The figure shows three views and two pictorial views of one solid part (mm, origin at its lowest corner). Answer the questions. A direction names the side the tool comes from. Give positions to 0.01 mm unless a question says otherwise; leave off trailing zeros. Write each loop counter-clockwise with the first axis right and the second up, starting at its lowest first coordinate (ties: lowest second). Pieces come first, ordered by that corner, then holes. Notation, with made-up numbers: M -35.5,-19.5 L -25.5,-19.5 A24 cw -25.5,18.5 Z; hole C 60,41 d1. An arc over 180 degrees is marked long. Answer as CSV lines item,"result". Start each with the question number.
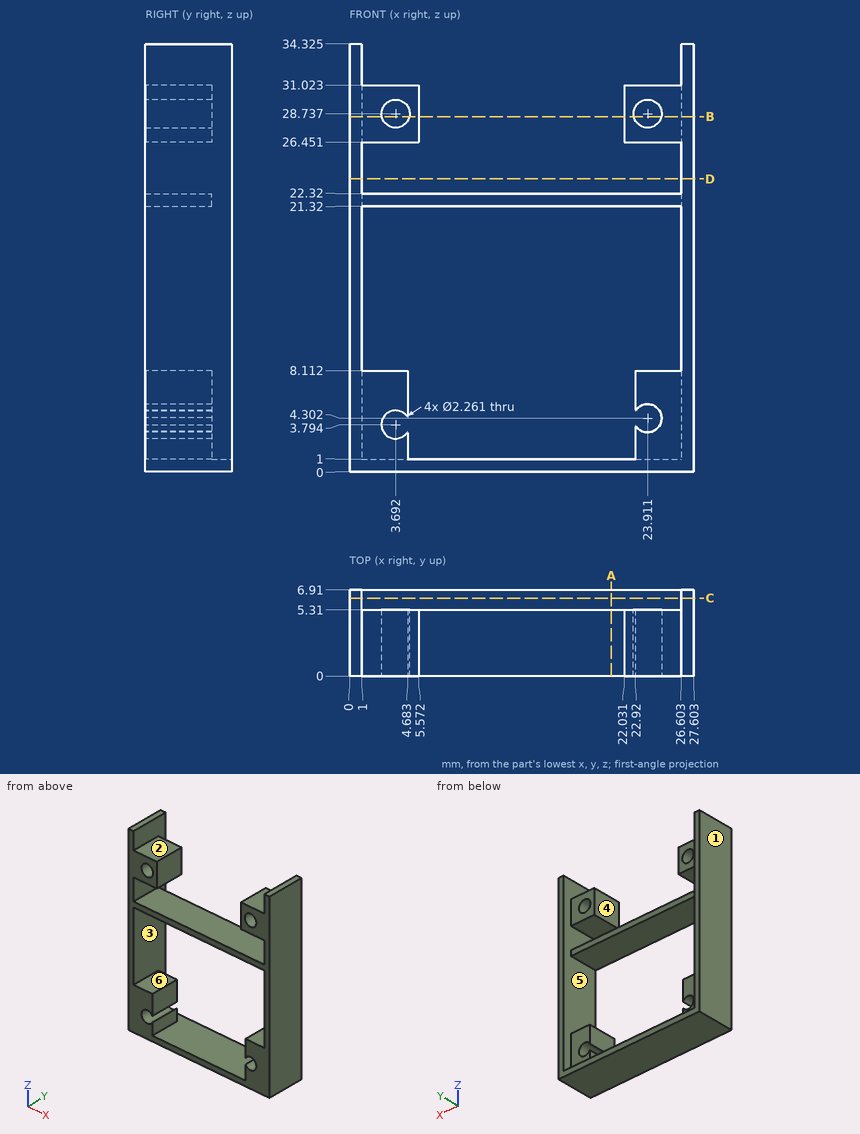
1. For the marked faces 4, 5 and 6, determine the directions among +Z, -Z, +X, -X, +Y, -Y from which every point of the face is accessible in a straight line to the end or side of a thin tool.
2. Find the intervals of material crossed by line 1 (Z direction, x = 17, y = 3); line 2 (X direction, y = 5.5, z = 22.5); line 3 (X direction, y = 1.25, z = 28.5) (1 decimal), in increasing order. Write a range as [from, to].
3. Given pin 1 (1.1 mm diameter, centred on x = 3.5, z = 5, fed in from +Y); pin 2 (1.1 mm diameter, centred on x = 2.5, y = 2, fed in from +Z); pin 3 (1 mm diameter, centred on x = 7.5, y = 5, fed in from +Z), each flat-ended and moving along its own axis, determine where each tip first touches the part or whether it passes through.
4. Find section C-C on y = 6.25. Determine the outline of the cut face in (x, z) (1 decimal).
5. Find section B-B on z = 28.5. Determine the outline of the cut face in (x, y) (1 decimal).
6. Find section D-D on z = 23.5. Determine the outline of the cut face in (x, y), then the cut area to 3 significant figures.
7. Find section A-A on x = 21. Determine the outline of the cut face in (y, z), then the cut area to 3 significant figures.
8. Determine the mould class of the marked faces 1, 2 and 3 for opening direction Z: +Z half, -Z half, draft (parallel to the pull), parting line (faces both ways), or undercut.
Computed:
1,face 4,"+Z, +Y, -Y"
1,face 5,"+Y"
1,face 6,"+Y, -Y"
2,line 1,"z = [0, 1], [21.32, 22.32]"
2,line 2,"x = [0, 1], [26.6, 27.6]"
2,line 3,"x = [0, 2.6], [4.8, 5.6], [22, 22.8], [25, 27.6]"
3,pin 1,"stops at y = 5.31"
3,pin 2,"stops at z = 31.02"
3,pin 3,"stops at z = 22.32"
4,outline,"M 0,0 L 27.6,0 L 27.6,34.3 L 26.6,34.3 L 26.6,1 L 1,1 L 1,34.3 L 0,34.3 Z"
5,outline,"M 0,0 L 2.6,0 L 2.6,5.3 L 1,5.3 L 1,6.9 L 0,6.9 Z; M 4.8,0 L 5.6,0 L 5.6,5.3 L 4.8,5.3 Z; M 22,0 L 22.8,0 L 22.8,5.3 L 22,5.3 Z; M 25,0 L 27.6,0 L 27.6,6.9 L 26.6,6.9 L 26.6,5.3 L 25,5.3 Z"
6,outline,"M 0,0 L 1,0 L 1,6.91 L 0,6.91 Z; M 26.6,0 L 27.6,0 L 27.6,6.91 L 26.6,6.91 Z"
6,area,"13.8 mm^2"
7,outline,"M 0,0 L 6.91,0 L 6.91,1 L 0,1 Z; M 0,21.32 L 5.31,21.32 L 5.31,22.32 L 0,22.32 Z"
7,area,"12.2 mm^2"
8,face 1,"draft"
8,face 2,"+Z half"
8,face 3,"undercut"
